Geometry: see drawing. Coordinates: mm, zero at the bounding-box minimum. A direction names the side the tool comes from. Give positions to 0.01 mm unless a question says otherwise; leave off trailing zeros. Write each loop counter-clockwise with the first axis right and the second up, starting at its lowest first coordinate (ties: lowest second). Pieces come first, ordered by that corner, then holes. Notation, with made-up numbers: M 11,-22 L 62,-22 A29 cw 62,9 Z; hole C -7.75,52 d9. An arc over 180 degrees is marked long. Use a Markdown table: item, result. Add a question column.
(1) Material intervals for L1, parallel to X at y = 10.75, z = 2.7; L2, parallel to X at y = 11.25, z = 2.6; L3, parallel to Z at x = 39.5, y = 15.5, sorted ascending.
(2) Pin query (flat end, axial travel): pin 1 Ø7 at (x, y) = (95, 10) entering from -Z; pin 2 Ø4.5 at (x, y) = (43, 17) entering from -Z. Return the tip coordinate at first contact, or that it passes through.
(3) Reachability of the marked faces 1, 2 and 3 from +Z, -Z, +X, -X, +Y, -Y: full face, straight path, thin tool, end or side. Return the list, or none.
(4) Cut plane D-D (x = 17). Output: boundary loops of the cut face in (y, z).
(5) Cut plane A-A (x = 73.75). Output: boundary loops of the cut face in (y, z), plus the area to 3 significant figures.
(6) Cut plane B-B (z = 2.3). Output: boundary loops of the cut face in (x, y).
(7) Cut plane C-C (y = 10). Output: boundary loops of the cut face in (x, z), plus the area to 3 significant figures.
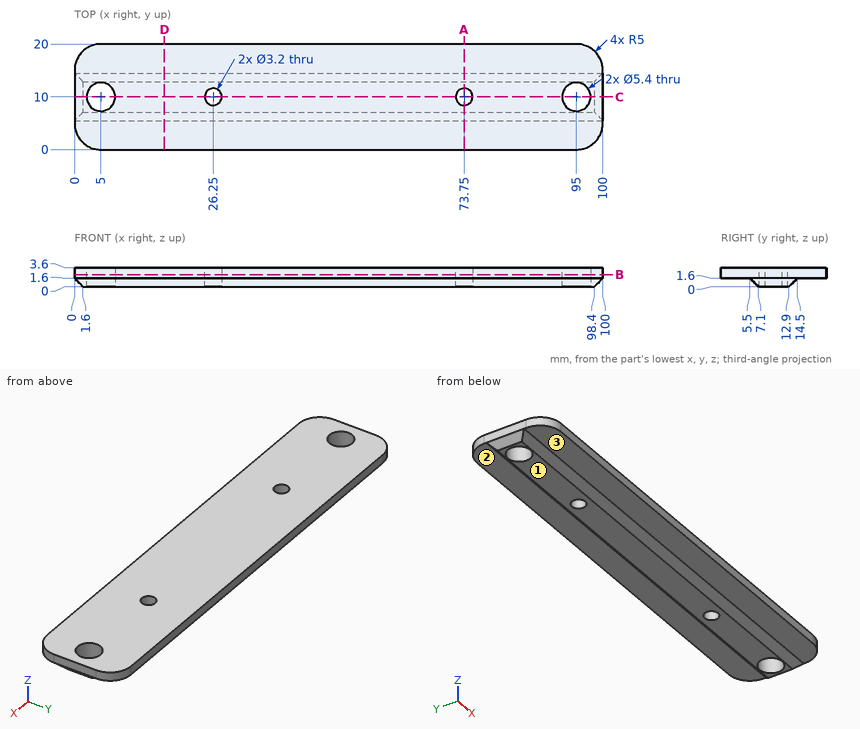
Answer list:
| question | item | result |
|---|---|---|
| 1 | L1 | 0 to 2.41, 7.59 to 24.84, 27.66 to 72.34, 75.16 to 92.41, 97.59 to 100 |
| 1 | L2 | 0 to 2.61, 7.39 to 25.25, 27.25 to 72.75, 74.75 to 92.61, 97.39 to 100 |
| 1 | L3 | 1.6 to 3.6 |
| 2 | pin 1 | z = 0 |
| 2 | pin 2 | z = 1.6 |
| 3 | face 1 | -Z, +X, -X, +Y, -Y |
| 3 | face 2 | -Z, +X, -X, +Y |
| 3 | face 3 | -Z, +X, -X, -Y |
| 4 | outline | M 0,1.6 L 5.5,1.6 L 7.1,0 L 12.9,0 L 14.5,1.6 L 20,1.6 L 20,3.6 L 0,3.6 Z |
| 5 | outline | M 0,1.6 L 5.5,1.6 L 7.1,0 L 8.4,0 L 8.4,3.6 L 0,3.6 Z; M 11.6,0 L 12.9,0 L 14.5,1.6 L 20,1.6 L 20,3.6 L 11.6,3.6 Z |
| 5 | area | 40.3 mm² |
| 6 | outline | M 0,5 A5 ccw 5,0 L 95,0 A5 ccw 100,5 L 100,15 A5 ccw 95,20 L 5,20 A5 ccw 0,15 Z; hole C 5,10 d5.4; hole C 26.25,10 d3.2; hole C 73.75,10 d3.2; hole C 95,10 d5.4 |
| 7 | outline | M 0,1.6 L 1.6,0 L 2.3,0 L 2.3,3.6 L 0,3.6 Z; M 7.7,0 L 24.65,0 L 24.65,3.6 L 7.7,3.6 Z; M 27.85,0 L 72.15,0 L 72.15,3.6 L 27.85,3.6 Z; M 75.35,0 L 92.3,0 L 92.3,3.6 L 75.35,3.6 Z; M 97.7,0 L 98.4,0 L 100,1.6 L 100,3.6 L 97.7,3.6 Z |
| 7 | area | 296 mm² |
